Input: part model. Units: mm. Frame: model coordinates. A direction names the side the tool comes from. Give positions to 0.01 mm unless a question says otherwise; leave off trailing zeros. Loops run counter-clockwise (first coordinate to the right, second up) from the corner with the lowest first, then second, coordinate; pieces in that order, holes last. Notation, with made-up numbers: (61.5, 65) -> (101.5, 65) arc R15 ccw to (101.5, 86) -> close; hole circle Ø11 at (56, 13.5). An arc over 180 degrees is marked (long way). Answer as a JSON object with one key per item and string values.
```python
from build123d import *

# Parameters (mm, degrees)
SKETCH1_W               = 60
SKETCH1_H               = 35
SKETCH1_W_2             = 46
SKETCH1_H_2             = 23
BOSS_EXTRUDE1_DEPTH     = 73
SKETCH2_W               = 46
SKETCH2_H               = 23
BOSS_EXTRUDE2_DEPTH     = 3
SKETCH1_3_R             = 2
CUT_EXTRUDE1_DEPTH      = 4.8
FILLET1_R               = 3
SKETCH3_W               = 46
SKETCH3_H               = 2.5
CUT_EXTRUDE2_DEPTH      = 1.1
SKETCH5_W               = 33
SKETCH5_H               = 42
CUT_EXTRUDE5_DEPTH      = 10
SKETCH5_3_W             = 35
SKETCH5_3_H             = 44
SKETCH5_3_W_2           = 33
SKETCH5_3_H_2           = 42
CUT_EXTRUDE6_DEPTH      = 2
CUT_EXTRUDE8_DEPTH      = 0.5
CUT_EXTRUDE8_DEPTH_BACK = 4.5
CUT_EXTRUDE9_DEPTH      = 0.5
CUT_EXTRUDE9_DEPTH_BACK = 4.5


with BuildPart() as part:
    # Sketch1 → Boss-Extrude1 (new body)
    with BuildSketch(Plane(origin=(0, 0, 0), x_dir=(0, 0, -1), z_dir=(1, 0, 0))):
        Rectangle(SKETCH1_W, SKETCH1_H)
        Rectangle(SKETCH1_W_2, SKETCH1_H_2, mode=Mode.SUBTRACT)
    extrude(amount=-BOSS_EXTRUDE1_DEPTH)

    # Sketch2 → Boss-Extrude2 (add)
    with BuildSketch(Plane.ZY.offset(73)):
        Rectangle(SKETCH2_W, SKETCH2_H)
    extrude(amount=-BOSS_EXTRUDE2_DEPTH)

    # Sketch1<3> → Cut-Extrude1 (cut)
    with BuildSketch(Plane(origin=(0, 0, 0), x_dir=(0, 0, -1), z_dir=(1, 0, 0))):
        with Locations((-26, 13.5)):
            Circle(SKETCH1_3_R)
        with Locations((0, 14.5)):
            Circle(SKETCH1_3_R)
        with Locations((26, 13.5)):
            Circle(SKETCH1_3_R)
        with Locations((0, -14.5)):
            Circle(SKETCH1_3_R)
        with Locations((-26, -13.5)):
            Circle(SKETCH1_3_R)
        with Locations((26, -13.5)):
            Circle(SKETCH1_3_R)
    extrude(amount=-CUT_EXTRUDE1_DEPTH, mode=Mode.SUBTRACT)

    # Fillet1
    fillet1_edges = [part.edges().sort_by_distance(p)[0] for p in [
        (-73, 17.5, 0),
        (-73, 0, 30),
        (-73, -17.5, 0),
        (-73, 0, -30),
        (-36.5, -17.5, 30),
        (-36.5, 17.5, 30),
        (-36.5, 17.5, -30),
        (-36.5, -17.5, -30),
    ]]
    fillet(fillet1_edges, radius=FILLET1_R)

    # Sketch3 → Cut-Extrude2 (cut)
    with BuildSketch(Plane(origin=(-70, 0, 0), x_dir=(0, 0, -1), z_dir=(1, 0, 0))):
        with Locations((0, -5.25)):
            Rectangle(SKETCH3_W, SKETCH3_H)
    extrude(amount=-CUT_EXTRUDE2_DEPTH, mode=Mode.SUBTRACT)

    # Sketch5 → Cut-Extrude5 (cut)
    with BuildSketch(Plane(origin=(0, 17.5, 0), x_dir=(1, 0, 0), z_dir=(0, 1, 0))):
        with Locations((-37.5, 0)):
            Rectangle(SKETCH5_W, SKETCH5_H)
    extrude(amount=-CUT_EXTRUDE5_DEPTH, mode=Mode.SUBTRACT)

    # Sketch5<3> → Cut-Extrude6 (cut)
    with BuildSketch(Plane(origin=(0, 17.5, 0), x_dir=(1, 0, 0), z_dir=(0, 1, 0))):
        with Locations((-37.5, 0)):
            Rectangle(SKETCH5_3_W, SKETCH5_3_H)
        with Locations((-37.5, 0)):
            Rectangle(SKETCH5_3_W_2, SKETCH5_3_H_2, mode=Mode.SUBTRACT)
    extrude(amount=-CUT_EXTRUDE6_DEPTH, mode=Mode.SUBTRACT)

    # Sketch7 → Cut-Extrude8 (cut, two sides)
    with BuildSketch(Plane.XY.offset(12.159)) as cut_extrude8_sk:
        Polygon((0, -11), (0, -14.307106781), (-3.307106781, -11), align=None)
    extrude(amount=CUT_EXTRUDE8_DEPTH, mode=Mode.SUBTRACT)
    extrude(cut_extrude8_sk.sketch, amount=-CUT_EXTRUDE8_DEPTH_BACK, mode=Mode.SUBTRACT)

    # Sketch8 → Cut-Extrude9 (cut, two sides)
    with BuildSketch(Plane(origin=(0, 0, -12.345376068), x_dir=(-1, 0, 0), z_dir=(0, 0, -1))) as cut_extrude9_sk:
        Polygon((0, -11), (3.307106781, -11), (0, -14.307106781), align=None)
    extrude(amount=CUT_EXTRUDE9_DEPTH, mode=Mode.SUBTRACT)
    extrude(cut_extrude9_sk.sketch, amount=-CUT_EXTRUDE9_DEPTH_BACK, mode=Mode.SUBTRACT)


solid = part.part
```
Q1. Draft query along Y for faces 1 (the flat face through (-73, 0, 0)), 2 (the flat face through (-1, -13, 12.659)), 3 (the cylindrical face through (-72.14, 16.6, -0.38)). Return one class per face: +Y half, -Y half, draft (parallel to the pull), parting line (faces both ways), or undercut.
Evaluation:
{"face 1": "draft", "face 2": "undercut", "face 3": "+Y half"}
Q2. Section B-B, the plane x = -56. Return the cut outline in (y, z), then the cut area to 3 significant figures.
Evaluation:
{"outline": "(-17.5, -27) arc R3 ccw to (-14.5, -30) -> (14.5, -30) arc R3 ccw to (17.5, -27) -> (17.5, 27) arc R3 ccw to (14.5, 30) -> (-14.5, 30) arc R3 ccw to (-17.5, 27) -> close; hole (-11.5, -23) -> (11.5, -23) -> (11.5, 23) -> (-11.5, 23) -> close", "area": "1,030 mm2"}
Q3. Pin query (flat end, axial travel): pin 1 (0.6 mm diameter, centred on y = 16.5, z = -11, fed in from -X); pin 2 (4 mm diameter, centred on y = -4, z = 12, fed in from +X); pin 3 (2.5 mm diameter, centred on y = -14.5, z = 0, fed in from +X). Return the tip coordinate at first contact, or that it passes through.
Evaluation:
{"pin 1": "stops at x = -72.47", "pin 2": "stops at x = -70", "pin 3": "stops at x = -4.8"}
Q4. Access query for faces 4 (the flat face through (0, 12, 0)), 5 (the flat face through (-4.8, 15, 0)), 6 (the flat face through (-54, 14, 0)). Directions: +Z, -Z, +X, -X, +Y, -Y. A direction counts if a zero-diameter tool reaches every point of the face in a straight line with its end or side. Return the directions, or none.
Evaluation:
{"face 4": "+Z, -Z, +X, +Y, -Y", "face 5": "+X", "face 6": "+Y"}
Q5. Section C-C, the plane y = -5.5. Return the cut outline in (x, z), then the cut area to 3 significant figures.
Evaluation:
{"outline": "(-73, -27) arc R3 ccw to (-70, -30) -> (0, -30) -> (0, -23) -> (-71.1, -23) -> (-71.1, 23) -> (0, 23) -> (0, 30) -> (-70, 30) arc R3 ccw to (-73, 27) -> close", "area": "1,110 mm2"}
Q6. Ray query, line 1 along Y through (x, z) = (-2.65, 0); line 2 along Y through (x, z) = (-2, -26); line 3 along Z through (x, y) = (-41, -2). Return the intervals inside material, ascending.
Evaluation:
{"line 1": "y = -17.5 to -16.5, -12.5 to -11.5, 11.5 to 12.5, 16.5 to 17.5", "line 2": "y = -17.5 to -15.5, -11.5 to 11.5, 15.5 to 17.5", "line 3": "z = -30 to -23, 23 to 30"}
Q7. Section D-D, the plane x = -34. Return the cut outline in (y, z), then the cut area to 3 significant figures.
Evaluation:
{"outline": "(-17.5, -27) arc R3 ccw to (-14.5, -30) -> (14.5, -30) arc R3 ccw to (17.5, -27) -> (17.5, -22) -> (15.5, -22) -> (15.5, -21) -> (11.5, -21) -> (11.5, -23) -> (-11.5, -23) -> (-11.5, 23) -> (11.5, 23) -> (11.5, 21) -> (15.5, 21) -> (15.5, 22) -> (17.5, 22) -> (17.5, 27) arc R3 ccw to (14.5, 30) -> (-14.5, 30) arc R3 ccw to (-17.5, 27) -> close", "area": "778 mm2"}
